from build123d import *

# Parameters (mm, degrees)
SKETCH_1_W          = 180
SKETCH_1_H          = 100
EXTRUDE_2_DEPTH     = 20
CUT_EXTRUDE_3_DEPTH = 2
CUT_EXTRUDE_4_DEPTH = 3.5
SKETCH_6_W          = 30
SKETCH_6_H          = 60
CUT_EXTRUDE_5_DEPTH = 50
MM_1_D              = 1
MM_1_DEPTH          = 4
MM_1_TIP            = 0.30043031


with BuildPart() as part:
    # 草图1 → 凸台-拉伸2 (new body)
    with BuildSketch(Plane(origin=(0, 0, 0), x_dir=(1, 0, 0), z_dir=(0, 1, 0))):
        with Locations((90, 50)):
            Rectangle(SKETCH_1_W, SKETCH_1_H)
    extrude(amount=EXTRUDE_2_DEPTH)

    # 草图4 → 切除-拉伸3 (cut)
    with BuildSketch(Plane(origin=(180, 0, 0), x_dir=(0, 0, -1), z_dir=(1, 0, 0))):
        with BuildLine():
            Line((48.811881188, 15.881188119), (20, 13))
            ThreePointArc((20, 13), (17, 10), (20, 7))
            Line((20, 7), (48.811881188, 4.118811881))
            ThreePointArc((48.811881188, 4.118811881), (50, 4), (51.188118812, 4.118811881))
            Line((51.188118812, 4.118811881), (80, 7))
            ThreePointArc((80, 7), (83, 10), (80, 13))
            Line((80, 13), (51.188118812, 15.881188119))
            ThreePointArc((51.188118812, 15.881188119), (50, 16), (48.811881188, 15.881188119))
        make_face()
    extrude(amount=-CUT_EXTRUDE_3_DEPTH, mode=Mode.SUBTRACT)

    # 草图5 → 切除-拉伸4 (cut)
    with BuildSketch(Plane(origin=(180, 0, 0), x_dir=(0, 0, -1), z_dir=(1, 0, 0))):
        Polygon((50, 16), (39.552109503, 14.95521095), (39.552109503, 5.04478905), (50, 4), (60.447890497, 5.04478905), (60.447890497, 14.95521095), align=None)
    extrude(amount=-CUT_EXTRUDE_4_DEPTH, mode=Mode.SUBTRACT)

    # 草图6 → 切除-拉伸5 (cut)
    with BuildSketch(Plane(origin=(0, 20, 0), x_dir=(1, 0, 0), z_dir=(0, 1, 0))):
        with Locations((160, 50)):
            Rectangle(SKETCH_6_W, SKETCH_6_H)
    extrude(amount=-CUT_EXTRUDE_5_DEPTH, mode=Mode.SUBTRACT)

    # 大小mm 暗销孔1
    with Locations(Plane(origin=(176.5, 9.952512246, -49.877349569), x_dir=(0, 0, 1), z_dir=(1, 0, 0))):
        with Locations((0, 0)):
            Hole(MM_1_D / 2, depth=MM_1_DEPTH)
            with Locations((0, 0, -(MM_1_DEPTH + MM_1_TIP / 2))):  # 118° drill point
                Cone(0, MM_1_D / 2, MM_1_TIP, mode=Mode.SUBTRACT)


solid = part.part
Geometry check sheet. Reference: the model listing, model coordinates, mm. A direction names the side the tool comes from. Give positions to 0.01 mm unless a question says otherwise; leave off trailing zeros. Write each loop counter-clockwise with the first axis right and the second up, starting at its lowest first coordinate (ties: lowest second). Pieces come first, ordered by that corner, then holes.
1) Thickness scan on line 1 (Z direction, x = 148, y = 9.25); line 2 (X direction, y = 11.5, z = -54); line 3 (X direction, y = 18.25, z = -69). Record the ranges inside material, lowest first.
Values follow:
line 1: z = -100 to -80, -20 to 0
line 2: x = 0 to 145, 175 to 176.5
line 3: x = 0 to 145, 175 to 180
2) Cross-section at B-B (x = 165). Record the boundary of the cut face in (y, z), plus the area to 3 significant figures.
Values follow:
outline: (0, -100) - (20, -100) - (20, -80) - (0, -80) - close; (0, -20) - (20, -20) - (20, 0) - (0, 0) - close
area: 800 mm2
3) Go/stop test with flat-tipped pins: pin 1 Ø6 at (y, z) = (13.5, -51) entering from +X; pin 2 Ø9.5 at (y, z) = (9.5, -47.5) entering from +X; pin 3 Ø5 at (y, z) = (8.5, -31) entering from +X. Record where each tip stops, or that it passes through.
Values follow:
pin 1: stops at x = 180
pin 2: stops at x = 176.5
pin 3: stops at x = 178
4) Cross-section at A-A (z = -55). Record the boundary of the cut face in (x, y), plus the area to 3 significant figures.
Values follow:
outline: (0, 0) - (145, 0) - (145, 20) - (0, 20) - close; (175, 0) - (180, 0) - (180, 4.5) - (176.5, 4.5) - (176.5, 15.5) - (180, 15.5) - (180, 20) - (175, 20) - close
area: 2,960 mm2
5) Release check for a two-part mould opening along Y. For faces 4 (the face through (176.5, 9, -50)), 5 (the face through (89, 20, -51)), 6 (the face through (178, 10, -28)), 7 (the face through (89, 10, -100)) record: released by +Y, released by -Y, zero draft, split by the parting line, or undercut.
Values follow:
face 4: undercut
face 5: released by +Y
face 6: undercut
face 7: zero draft
6) Cross-section at C-C (y = 18). Record the boundary of the cut face in (x, z), plus the area to 3 significant figures.
Values follow:
outline: (0, -100) - (180, -100) - (180, 0) - (0, 0) - close; hole (145, -80) - (175, -80) - (175, -20) - (145, -20) - close
area: 16,200 mm2
7) Set-up check for faces 1 (the face through (0, 10, -49)), 2 (the face through (178, 10, -69)), 3 (the face through (145, 10, -50)): record each of +Z, -Z, +X, -X, +Y, -Y from which the full face is reachable in a straight line by a thin tool's end or side.
Values follow:
face 1: +Z, -Z, -X, +Y, -Y
face 2: +X
face 3: +Y, -Y
